Geometry: see drawing. Coordinates: mm, zero at the bounding-box minimum. Give positions to 0.01 mm unless a question says otherwise; leave off trailing zeros. Order: outer loops, then holes, each group sorted by start corner. A loop starts at its lowest first (then second) coordinate and runs counter-clockwise, first axis right, second up. Notation, with made-up numbers: M 24,54.25 L 31,54.25 A16 cw 31,63.25 Z; hole C -6.5,-34 d2. An arc over 180 degrees is marked long. Return JSON: item names as keys, results as strings.
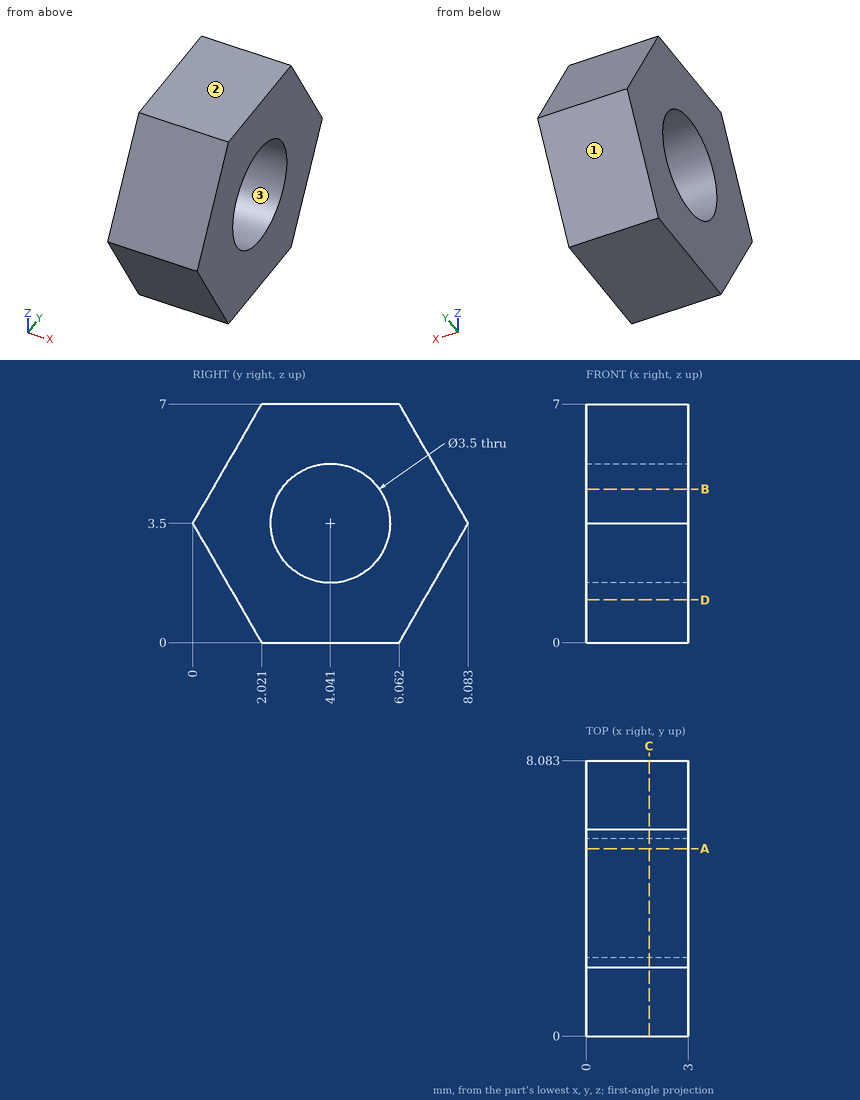
1. Section query C-C (x = 1.85). Return loops of the section in (y, z).
Evaluation:
{"outline": "M 0,3.5 L 2.02,0 L 6.06,0 L 8.08,3.5 L 6.06,7 L 2.02,7 Z; hole C 4.04,3.5 d3.5"}
2. Draft query along Y for the marked faces 1, 2 and 3. Return one class per face: pulls with the +Y half, pulls with the -Y half, needs draft (parallel to the pull), parting line crosses it, or undercut.
Evaluation:
{"face 1": "pulls with the +Y half", "face 2": "needs draft", "face 3": "undercut"}
3. First-contact query: pin 1 (1.5 mm diameter, centred on x = 1, z = 5, fed in from -Y). Flat tip, straight axial feed; report the tip coordinate or a pass-through.
Evaluation:
{"pin 1": "stops at y = 0.43"}
4. Section query D-D (z = 1.25). Return loops of the section in (x, y).
Evaluation:
{"outline": "M 0,1.3 L 3,1.3 L 3,6.78 L 0,6.78 Z"}
5. Section query B-B (z = 4.5). Return loops of the section in (x, y) (1 decimal).
Evaluation:
{"outline": "M 0,0.6 L 3,0.6 L 3,2.6 L 0,2.6 Z; M 0,5.5 L 3,5.5 L 3,7.5 L 0,7.5 Z"}
6. Section query A-A (y = 5.5). Return loops of the section in (x, z), then the cut area to 3 significant figures.
Evaluation:
{"outline": "M 0,0 L 3,0 L 3,2.53 L 0,2.53 Z; M 0,4.47 L 3,4.47 L 3,7 L 0,7 Z", "area": "15.2 mm^2"}
7. Ray query, probe 1 along Z at (x, y) = (1.6, 3.5) (1 decimal); probe 2 along Y at (x, z) = (0.95, 2) (1 decimal); probe 3 along Y at (x, z) = (0.2, 3) (1 decimal). Return the intervals inside material, ascending.
Evaluation:
{"probe 1": "z = 0 to 1.8, 5.2 to 7", "probe 2": "y = 0.9 to 3.1, 4.9 to 7.2", "probe 3": "y = 0.3 to 2.4, 5.7 to 7.8"}
